Could you check a few things on this model? Use its own coordinates, in mm. Coordinates: 2 decimals unless noted, no trailing zeros. Loops run counter-clockwise (first coordinate to the right, second up) from the corner with the lowest first, then second, coordinate; pieces in that order, holes last. Notation, with made-up numbers: (31, 54.5) -> (85, 54.5) arc R17 ccw to (85, 82.5) -> close; hole circle Ø8 at (34, 5). An arc over 180 degrees is marked (long way). One line per question, with ' | ' between items. Start each with the question number.
(1) Suppose I cut it at A-A (y = 40). Please give me the cut outline in (x, z).
(2) If I drill on line 1 along Y through (x, z) = (20, 1.2); line 2 along Y through (x, z) = (0, 2.2); line 3 along Y through (x, z) = (-24, 2.65), over which ranges is the centre line in solid material (lowest first)?
(3) Suppose I cut it at C-C (x = 20). Please give me the cut outline in (y, z).
(4) Suppose I cut it at B-B (y = 0). Please give me the cut outline in (x, z), plus the area to 3 significant figures.
(5) Suppose I cut it at D-D (y = 20). Please give me the cut outline in (x, z), plus the area to 3 significant figures.
(6) I'm going to push flat-ended pins straight in: pin 1 Ø1.2 at (x, z) = (20.5, 1.5) entering from +Y; pin 2 Ø1.5 at (x, y) = (-5, 41.5) entering from -Z; pin 3 Ø2.5 at (x, y) = (-20, 40) entering from +Z (1 decimal); pin 4 Ø1.2 at (y, z) = (92, 1.5) entering from +X. Where does each tip first touch, or does it pass through?
```python
from build123d import *

# Parameters (mm, degrees)
SKETCH_1_R      = 4.5
SKETCH_1_R_2    = 2
EXTRUDE_1_DEPTH = 4


with BuildPart() as part:
    # 草图1 → 凸台-拉伸1 (new body)
    with BuildSketch(Plane.XY):
        Polygon((-39, 90), (-39, -46), (39, -46), (39, 90), (27.5, 90), (27.5, 86), (28.85, 86), (28.85, 83.3), (27.5, 83.3), (27.5, 81.3), (24.5, 81.3), (24.5, 83.3), (23.15, 83.3), (23.15, 86), (24.5, 86), (24.5, 90), (17, 90), (17, 94), (9, 94), (9, 90), (1.5, 90), (1.5, 86), (2.85, 86), (2.85, 83.3), (1.5, 83.3), (1.5, 81.3), (-1.5, 81.3), (-1.5, 83.3), (-2.85, 83.3), (-2.85, 86), (-1.5, 86), (-1.5, 90), (-9, 90), (-9, 94), (-17, 94), (-17, 90), (-24.5, 90), (-24.5, 86), (-23.15, 86), (-23.15, 83.3), (-24.5, 83.3), (-24.5, 81.3), (-27.5, 81.3), (-27.5, 83.3), (-28.85, 83.3), (-28.85, 86), (-27.5, 86), (-27.5, 90), align=None)
        Circle(SKETCH_1_R, mode=Mode.SUBTRACT)
        with Locations((20, 0)):
            Circle(SKETCH_1_R_2, mode=Mode.SUBTRACT)
        with Locations((0, 20)):
            Circle(SKETCH_1_R_2, mode=Mode.SUBTRACT)
        with Locations((-20, 40)):
            Circle(SKETCH_1_R_2, mode=Mode.SUBTRACT)
        with Locations((-20, 0)):
            Circle(SKETCH_1_R_2, mode=Mode.SUBTRACT)
        with Locations((20, 40)):
            Circle(SKETCH_1_R_2, mode=Mode.SUBTRACT)
    extrude(amount=EXTRUDE_1_DEPTH)


solid = part.part
```
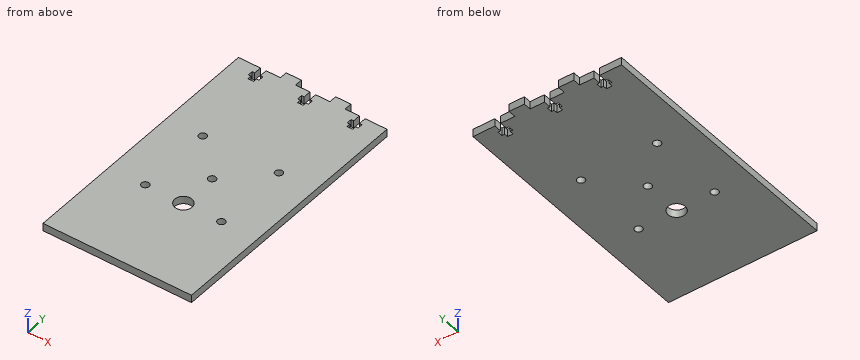
Checks:
1) outline: (-39, 0) -> (-22, 0) -> (-22, 4) -> (-39, 4) -> close; (-18, 0) -> (18, 0) -> (18, 4) -> (-18, 4) -> close; (22, 0) -> (39, 0) -> (39, 4) -> (22, 4) -> close
2) line 1: y = -46 to -2, 2 to 38, 42 to 90 | line 2: y = -46 to -4.5, 4.5 to 18, 22 to 81.3 | line 3: y = -46 to 83.3, 86 to 90
3) outline: (-46, 0) -> (-2, 0) -> (-2, 4) -> (-46, 4) -> close; (2, 0) -> (38, 0) -> (38, 4) -> (2, 4) -> close; (42, 0) -> (90, 0) -> (90, 4) -> (42, 4) -> close
4) outline: (-39, 0) -> (-22, 0) -> (-22, 4) -> (-39, 4) -> close; (-18, 0) -> (-4.5, 0) -> (-4.5, 4) -> (-18, 4) -> close; (4.5, 0) -> (18, 0) -> (18, 4) -> (4.5, 4) -> close; (22, 0) -> (39, 0) -> (39, 4) -> (22, 4) -> close | area: 244 mm^2
5) outline: (-39, 0) -> (-2, 0) -> (-2, 4) -> (-39, 4) -> close; (2, 0) -> (39, 0) -> (39, 4) -> (2, 4) -> close | area: 296 mm^2
6) pin 1: stops at y = 90 | pin 2: stops at z = 0 | pin 3: passes through | pin 4: stops at x = 17
